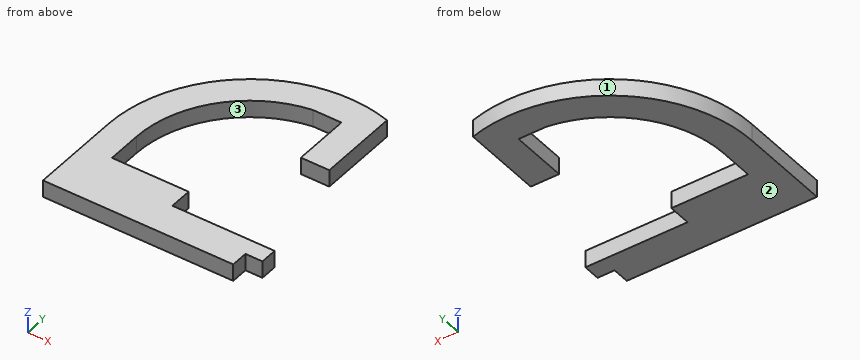
```python
from build123d import *

# Parameters (mm, degrees)
EXTRUDE_1_DEPTH = 6


with BuildPart() as part:
    # Эскиз2 → Бобышка-Вытянуть1 (new body)
    with BuildSketch(Plane.XY):
        with BuildLine():
            Line((10, 20), (10, 32))
            ThreePointArc((10, 32), (19.668498224, 58.076809621), (44, 71.547439867))
            Line((44, 71.547439867), (54, 71.547439867))
            Line((54, 71.547439867), (54, 51.547439867))
            Line((54, 51.547439867), (64, 51.547439867))
            Line((64, 51.547439867), (64, 80))
            ThreePointArc((64, 80), (20, 72), (0, 32))
            Line((0, 32), (0, 0))
            Line((0, 0), (67, 0))
            Line((67, 0), (67, 6))
            Line((67, 6), (73, 6))
            Line((73, 6), (73, 12))
            Line((73, 12), (67, 12))
            Line((67, 12), (37, 12))
            Line((37, 12), (37, 20))
            Line((37, 20), (10, 20))
        make_face()
    extrude(amount=EXTRUDE_1_DEPTH)


solid = part.part
```
For this review, take the finished solid that the model builds, in its own axes (mm). Face numbers are marked on the shaded views. Give positions to 0.01 mm unless a question says otherwise; leave off trailing zeros. Write each loop counter-clockwise with the first axis right and the second up, starting at its lowest first coordinate (ties: lowest second). Pieces come first, ordered by that corner, then holes. Notation, with made-up numbers: M 23,66.25 L 28,66.25 A37 ccw 28,104.25 Z; hole C 5,67.25 d7. An arc over 180 degrees is marked long. One line per item, written item: value.
1) For P1, Ø3, axis at y = 56, z = 4.5, coming from the -X side; P2, Ø3, axis at y = 70, z = 3.5, coming from the +X side; P3, Ø3, axis at y = 15.5, z = 3, coming from the +X side; P4, Ø1, axis at y = 21, z = 1, coming from the -X side, all flat-tipped, find the tip position at first contact; note any pin that passes through.
Results are:
P1: stops at x = 5.35
P2: stops at x = 64
P3: stops at x = 37
P4: stops at x = 0
2) Take a section at C-C, the plane y = 67.5. Write out the cut boundary in (x, z).
Results are:
outline: M 14.79,0 L 31.57,0 L 31.57,6 L 14.79,6 Z; M 54,0 L 64,0 L 64,6 L 54,6 Z
3) Take a section at B-B, the plane z = 2.55. Write out the cut boundary in (x, y), then the cut area to 3 significant figures.
Results are:
outline: M 0,0 L 67,0 L 67,6 L 73,6 L 73,12 L 37,12 L 37,20 L 10,20 L 10,32 A40 cw 44,71.55 L 54,71.55 L 54,51.55 L 64,51.55 L 64,80 A50 ccw 0,32 Z
area: 2,300 mm²
4) Take a section at D-D, the plane y = 15.5. Write out the cut boundary in (x, z), then the cut area to 3 significant figures.
Results are:
outline: M 0,0 L 37,0 L 37,6 L 0,6 Z
area: 222 mm²
5) Take a section at A-A, the plane x = 48. Write out the cut boundary in (y, z).
Results are:
outline: M 0,0 L 12,0 L 12,6 L 0,6 Z; M 71.55,0 L 81.96,0 L 81.96,6 L 71.55,6 Z
6) The part is to be moulded in two halves that separate along X. For the marked faces 1, 2 and 3, say which applies: +X half, -X half, draft (parallel to the pull), parting line (faces both ways), or undercut.
Results are:
face 1: parting line
face 2: draft
face 3: undercut
7) For line 1 (X direction, y = 19, z = 2.4); line 2 (Y direction, x = 41, z = 5.35); line 3 (Y direction, x = 43, z = 2.5), list the stretches that pass through material, from the lowest coordinate up. Write a range as from..to.
Results are:
line 1: x = 0..37
line 2: y = 0..12, 70.97..81.18
line 3: y = 0..12, 71.38..81.51
